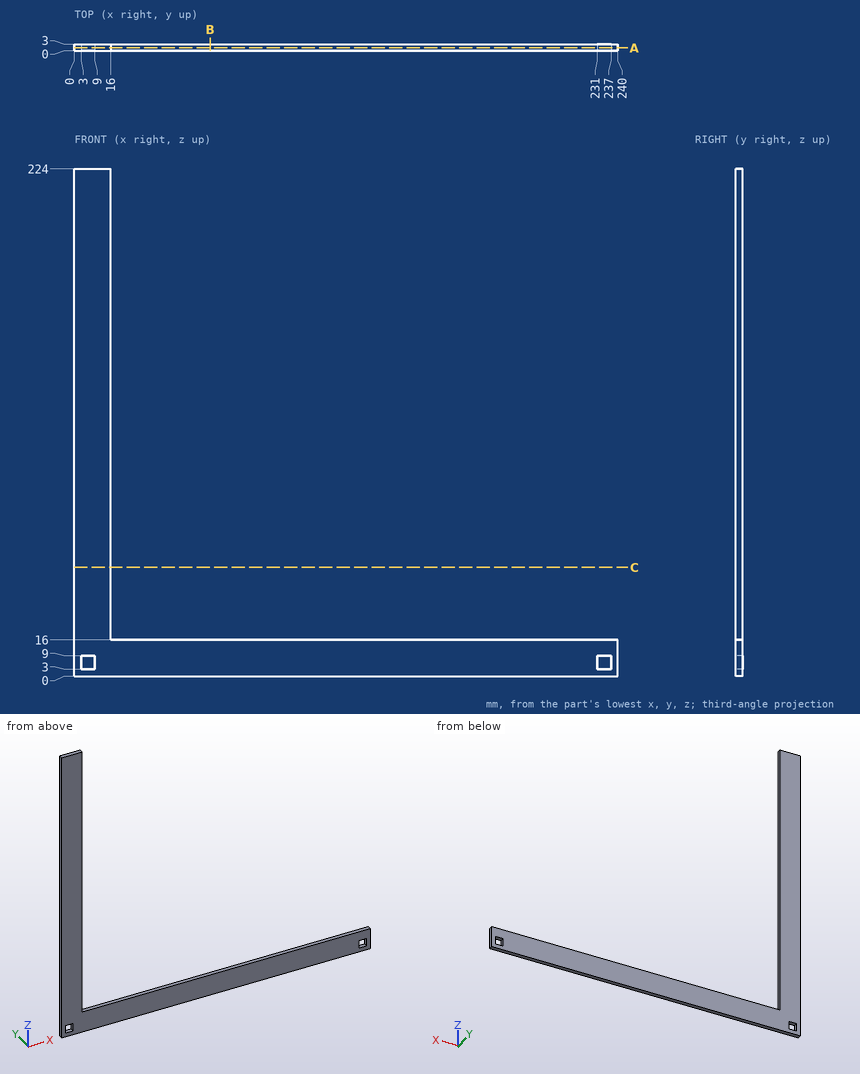
The drawing under review shows one solid part. Ordinate dimensions are in mm from its lowest x, y, z. Coordinates: 2 decimals unless noted, no trailing zeros. Write each loop counter-clockwise with the first axis right and the second up, starting at its lowest first coordinate (ties: lowest second). Pieces come first, ordered by that corner, then holes. Notation, with made-up numbers: (-27.5, 64) -> (22.5, 64) arc R20 ccw to (22.5, 95) -> close; hole circle Ø1 at (75, 21). An arc over 180 degrees is marked (long way). One line per item, written item: value. Start each with the question number.
Q1. To check wall thickness, follow probe 1 along X at (y, z) = (2.8, 125). State the ranges of the line that lie inside material, in increasing order.
Q2. Add section A-A, the plane y = 1.3. Give the boundary of the cut face in (x, z), then the cut area to 3 significant figures.
Q3. Add section C-C, the plane z = 48. Give the boundary of the cut face in (x, y).
Q4. Clearance check with flat-ended pins moving along their axes: P1, Ø1.5, axis at y = 1.5, z = 142.5, coming from the +X side; P2, Ø0.9, axis at x = 111.5, y = 1, coming from the +Z side. State where each tip first meets the part, or that it passes through.
Q5. Add section B-B, the plane x = 60. Give the boundary of the cut face in (y, z).
Response:
1. probe 1: 0 to 16
2. outline: (0, 0) -> (240, 0) -> (240, 16) -> (16, 16) -> (16, 224) -> (0, 224) -> close; hole (3, 3) -> (9, 3) -> (9, 9) -> (3, 9) -> close; hole (231, 3) -> (237, 3) -> (237, 9) -> (231, 9) -> close
2. area: 7,100 mm²
3. outline: (0, 0) -> (16, 0) -> (16, 3) -> (0, 3) -> close
4. P1: x = 16
4. P2: z = 16
5. outline: (0, 0) -> (3, 0) -> (3, 16) -> (0, 16) -> close
